```python
from build123d import *

# Parameters (mm, degrees)
F1_DEPTH = 12
F3_R     = 16
F4_DEPTH = 12.001
F5_R     = 17
F5_R_2   = 16
F6_DEPTH = 2
F2_R     = 17
F7_DEPTH = 9


# Not quite as in the source:
# - the program builds the solid bodies; features that only make, move or delete a surface that nothing else refers to are left out


with BuildPart() as f1:
    # F0 (on Top) → F1 (new body)
    with BuildSketch(Plane.XY):
        with BuildLine():
            Line((10.5367190596, 20), (0, 20))
            Line((0, 20), (-10, 20))
            ThreePointArc((-10, 20), (-10.7071067812, 20.2928932188), (-11, 21))
            Line((-11, 21), (-11, 26))
            Line((-11, 26), (-13.1087498209, 26))
            ThreePointArc((-13.1087498209, 26), (-13.7740978096, 25.7465333576), (-14.1021587568, 25.114624108))
            Line((-14.1021587568, 25.114624108), (-14.5904720191, 20.8825758343))
            ThreePointArc((-14.5904720191, 20.8825758343), (-15.8474732978, 14.5432941931), (-18.1089431513, 8.4891800512))
            ThreePointArc((-18.1089431513, 8.4891800512), (-20, 0), (-18.1089431513, -8.4891800512))
            ThreePointArc((-18.1089431513, -8.4891800512), (-15.8474732978, -14.5432941931), (-14.5904720191, -20.8825758343))
            Line((-14.5904720191, -20.8825758343), (-14.1021587568, -25.114624108))
            ThreePointArc((-14.1021587568, -25.114624108), (-13.7740978096, -25.7465333576), (-13.1087498209, -26))
            Line((-13.1087498209, -26), (-11, -26))
            Line((-11, -26), (-11, -21))
            ThreePointArc((-11, -21), (-10.7071067812, -20.2928932188), (-10, -20))
            Line((-10, -20), (0, -20))
            Line((0, -20), (10, -20))
            ThreePointArc((10, -20), (10.7071067812, -20.2928932188), (11, -21))
            Line((11, -21), (11, -26))
            Line((11, -26), (13.1087498209, -26))
            ThreePointArc((13.1087498209, -26), (13.7740978096, -25.7465333576), (14.1021587568, -25.114624108))
            Line((14.1021587568, -25.114624108), (14.5904720191, -20.8825758343))
            ThreePointArc((14.5904720191, -20.8825758343), (15.8474732978, -14.5432941931), (18.1089431513, -8.4891800512))
            ThreePointArc((18.1089431513, -8.4891800512), (20, 0), (18.1089431513, 8.4891800512))
            ThreePointArc((18.1089431513, 8.4891800512), (15.8474732978, 14.5432941931), (14.5904720191, 20.8825758343))
            Line((14.5904720191, 20.8825758343), (14.1021587568, 25.114624108))
            ThreePointArc((14.1021587568, 25.114624108), (13.7740978096, 25.7465333576), (13.1087498209, 26))
            Line((13.1087498209, 26), (11, 26))
            Line((11, 26), (11, 20.8437610154))
            ThreePointArc((11, 20.8437610154), (10.8765611957, 20.3624705935), (10.5367190596, 20))
        make_face()
    extrude(amount=F1_DEPTH)

    # F3 (on face) → F4 (cut, through all)
    with BuildSketch(Plane.XY.offset(12)):
        Circle(F3_R)
    extrude(amount=-F4_DEPTH, mode=Mode.SUBTRACT)

    # F5 (on face) → F6 (cut)
    with BuildSketch(Plane.XY.offset(12)):
        Circle(F5_R)
        Circle(F5_R_2, mode=Mode.SUBTRACT)
    extrude(amount=-F6_DEPTH, mode=Mode.SUBTRACT)

    # F2 (on face) → F7 (cut)
    with BuildSketch(Plane(origin=(0, 0, 0), x_dir=(1, 0, 0), z_dir=(0, 0, -1))):
        Circle(F2_R)
    extrude(amount=-F7_DEPTH, mode=Mode.SUBTRACT)


solid = f1.part
```
Build history of the part. All positions in model axes, mm. A direction names the side the tool comes from. Give positions to 0.01 mm unless a question says otherwise; leave off trailing zeros. Loops run counter-clockwise (first coordinate to the right, second up) from the corner with the lowest first, then second, coordinate; pieces in that order, holes last.
1) 3-axis set-ups, long thin cutter, end or side, ignore diameter. For faces 5 (the face through (-15.87, -14.46, 5.92)), 6 (the face through (0, 20, 6)), 7 (the face through (11, -23, 6)), 8 (the face through (9.139, 14.334, 11.014)): which of +Z, -Z, +X, -X, +Y, -Y reach the whole face in a straight line?
Values follow:
face 5: +Z, -Z, -X, -Y
face 6: +Z, -Z, +Y
face 7: +Z, -Z, -Y
face 8: +Z
2) Drop flat-ended pins along their axis: P1, Ø4, axis at y = -24.5, z = 9, coming from the -X side; P2, Ø5.5, axis at y = 23, z = 7, coming from the -X side; P3, Ø2.5, axis at y = 24.5, z = 5, coming from the +X side. Give the stop position or say it passes through.
Values follow:
P1: stops at x = -14.4
P2: stops at x = -14.67
P3: stops at x = 14.32
3) Two-plate mould, pull along Y, no slides. Class faces 1 (the face through (-14.35, -22.97, 5.92)), 2 (the face through (13, -10, 10)), 3 (the face through (9.139, -14.334, 4.437)), 4 (the face through (7, 16, 12)): released by +Y, released by -Y, zero draft, split by the parting line, or undercut.
Values follow:
face 1: released by -Y
face 2: undercut
face 3: undercut
face 4: zero draft
4) Band-saw the part on B-B on y = -1. List the corners of the cut face in (x, z).
Values follow:
outline: (-19.97, 0) - (-16.97, 0) - (-16.97, 9) - (-15.97, 9) - (-15.97, 10) - (-16.97, 10) - (-16.97, 12) - (-19.97, 12) - close; (15.97, 9) - (16.97, 9) - (16.97, 0) - (19.97, 0) - (19.97, 12) - (16.97, 12) - (16.97, 10) - (15.97, 10) - close
5) Band-saw the part on A-A on x = 0. List the corners of the cut face in (y, z), then the cut area to 3 significant figures.
Values follow:
outline: (-20, 0) - (-17, 0) - (-17, 9) - (-16, 9) - (-16, 10) - (-17, 10) - (-17, 12) - (-20, 12) - close; (16, 9) - (17, 9) - (17, 0) - (20, 0) - (20, 12) - (17, 12) - (17, 10) - (16, 10) - close
area: 74.0 mm2
6) Probe line 1 along Y through (x, z) = (0.5, 9.75); line 2 along Y through (x, z) = (0, 11.3); line 3 along Z through (x, y) = (15.5, 5). List the from-to ranges inside material, lowest first.
Values follow:
line 1: y = -20 to -15.99, 15.99 to 20
line 2: y = -20 to -17, 17 to 20
line 3: z = 9 to 10
